```python
from build123d import *

# Parameters (mm, degrees)
F1_DEPTH = 2.54
F2_R     = 2.53999


# Not quite as in the source:
# - a fillet or chamfer is up to 0.001 mm smaller than in the source, because OpenCascade refuses the exact size


with BuildPart() as f1:
    # F0 (on Top) → F1 (new body)
    with BuildSketch(Plane.XY):
        with BuildLine():
            ThreePointArc((0, -6.35), (4.4901280605, -4.4901280605), (6.35, 0))
            ThreePointArc((6.35, 0), (4.4901280605, 4.4901280605), (0, 6.35))
            ThreePointArc((0, 6.35), (-4.4901280605, 4.4901280605), (-6.35, 0))
            ThreePointArc((-6.35, 0), (-4.4901280605, -4.4901280605), (0, -6.35))
        make_face()
        with BuildLine():
            ThreePointArc((3.81, 0), (0, -3.81), (-3.81, 0))
            ThreePointArc((-3.81, 0), (0, 3.81), (3.81, 0))
        make_face(mode=Mode.SUBTRACT)
        with BuildLine():
            ThreePointArc((-6.35, 0), (-4.4901280605, 4.4901280605), (0, 6.35))
            Line((0, 6.35), (-6.35, 6.35))
            Line((-6.35, 6.35), (-6.35, 0))
        make_face()
        with BuildLine():
            Line((-6.35, -6.35), (0, -6.35))
            ThreePointArc((0, -6.35), (-4.4901280605, -4.4901280605), (-6.35, 0))
            Line((-6.35, 0), (-6.35, -6.35))
        make_face()
    extrude(amount=F1_DEPTH)

    # F2 (radius 2.54 in the source; OpenCascade refuses exactly that, so slightly less here)
    f2_edges = [f1.edges().sort_by_distance(p)[0] for p in [
        (-3.175, 6.35, 2.54),
    ]]
    fillet(f2_edges, radius=F2_R)


solid = f1.part
```
For this review, take the finished solid that the model builds, in its own axes (mm). Round coordinates to 2 decimals unless told otherwise and drop trailing zeros. Write each loop counter-clockwise with the first axis right and the second up, starting at its lowest first coordinate (ties: lowest second). Pieces come first, ordered by that corner, then holes. Notation, with made-up numbers: (-6, 69) - (27, 69) arc R8 cw to (27, 74) - close; hole circle Ø6 at (58, -19). An arc over 180 degrees is marked (long way). Answer as a JSON object with one key per item and string values.
1. For pin 1 Ø7 at (x, y) = (0, 0) entering from -Z, flat-tipped, find the tip position at first contact; note if it passes through.
Response values:
{"pin 1": "passes through"}
2. We need section B-B on z = 1.35. Give the boundary of the cut face in (x, y), then the cut area to 3 significant figures.
Response values:
{"outline": "(-6.35, -5.96) - (0, -5.96) arc R5.96 ccw to (0, 5.96) - (-6.35, 5.96) - close; hole circle Ø7.62 at (0, 0)", "area": "85.9 mm2"}
3. We need section D-D on z = 0.5. Give the boundary of the cut face in (x, y), then the cut area to 3 significant figures.
Response values:
{"outline": "(-6.35, -6.3) - (0, -6.3) arc R6.3 ccw to (0, 6.3) - (-6.35, 6.3) - close; hole circle Ø7.62 at (0, 0)", "area": "96.8 mm2"}
4. To check wall thickness, follow line 1 along Y through (x, z) = (0, 0.8); line 2 along X through (y, z) = (-2.5, 1.7); line 3 along X through (y, z) = (0.25, 1.2). State the ranges of each line that lie inside material, in increasing order.
Response values:
{"line 1": "y = -6.22 to -3.81, 3.81 to 6.22", "line 2": "x = -6.35 to -2.88, 2.88 to 5.12", "line 3": "x = -6.35 to -3.8, 3.8 to 6.04"}
5. Draft analysis for pull direction X (two halves, no side actions). For faces 1 (the face through (-6.35, 0, 1)), 2 (the face through (0.83, -3.72, 1.25)), 3 (the face through (-5, 0, 2.54)), state which applies: +X half, -X half, draft (parallel to the pull), parting line (faces both ways), or undercut.
Response values:
{"face 1": "-X half", "face 2": "undercut", "face 3": "draft"}
